Source: CAD feature listing. Evaluate the final solid. Frame: model axes, mm. Face numbers are marked on the shaded views. A direction names the side the tool comes from. Coordinates: 2 decimals unless noted, no trailing zeros. Order: outer loops, then holes, each group sorted by start corner. A loop starts at its lowest first (then second) coordinate and runs counter-clockwise, first axis right, second up.
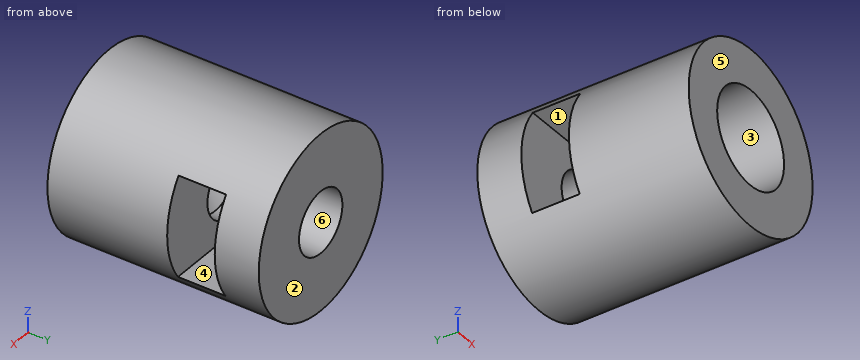
```python
from build123d import *

# Parameters (mm, degrees)
F3_R     = 5
F4_DEPTH = 12
F6_D     = 5.4
F6_DEPTH = 3
F6_TIP   = 1.6223236714
F7_D     = 3.5
F7_DEPTH = 6
F7_TIP   = 1.0515060833
F8_W     = 2.7
F8_H     = 5.7
F9_DEPTH = 38.4228628705


with BuildPart() as f4:
    # F3 (on Front) → F4 (new body)
    with BuildSketch(Plane.XZ):
        with Locations((-33.4218628705, 28.5066645592)):
            Circle(F3_R)
    extrude(amount=-F4_DEPTH)

    # F6
    with Locations(Plane.XZ):
        with Locations((-33.4218628705, 28.5066645592)):
            Hole(F6_D / 2, depth=F6_DEPTH)
            with Locations((0, 0, -(F6_DEPTH + F6_TIP / 2))):  # 118° drill point
                Cone(0, F6_D / 2, F6_TIP, mode=Mode.SUBTRACT)

    # F7
    with Locations(Plane(origin=(0, 12, 0), x_dir=(-1, 0, 0), z_dir=(0, 1, 0))):
        with Locations((33.4218628705, 28.5066645592)):
            Hole(F7_D / 2, depth=F7_DEPTH)
            with Locations((0, 0, -(F7_DEPTH + F7_TIP / 2))):  # 118° drill point
                Cone(0, F7_D / 2, F7_TIP, mode=Mode.SUBTRACT)

    # F8 (on Right) → F9 (cut, through all)
    with BuildSketch(Plane.YZ):
        with Locations((8.15, 28.5412482917)):
            Rectangle(F8_W, F8_H)
    extrude(amount=-F9_DEPTH, mode=Mode.SUBTRACT)


solid = f4.part
```
1. Ray query, line 1 (Z direction, x = -33.5, y = 10.5); line 2 (Y direction, x = -29.25, z = 29.25); line 3 (Z direction, x = -33.5, y = 8). Return the intervals inside material, ascending.
Findings:
line 1: z = 23.51 to 26.76, 30.25 to 33.51
line 2: y = 0 to 6.8, 9.5 to 12
line 3: z = 23.51 to 25.69, 31.39 to 33.51
2. Draft query along Y for the marked faces 4, 5 and 6. Return one class per face: released by +Y, released by -Y, zero draft, split by the parting line, or undercut.
Findings:
face 4: undercut
face 5: released by -Y
face 6: zero draft
3. Section query D-D on y = 11. Return loops of the section in (x, z), plus the area to 3 significant figures.
Findings:
outline: circle Ø10 at (-33.42, 28.51); hole circle Ø3.5 at (-33.42, 28.51)
area: 68.9 mm2
4. Section query C-C on z = 29.25. Count the separate pieces of the cut face and the enclosed holes in it, plus the area to 3 significant figures.
Findings:
separate pieces: 3
enclosed holes: 0
area: 61.2 mm2
5. Access query for the marked faces 1, 2 and 3. Directions: +Z, -Z, +X, -X, +Y, -Y. A direction counts if a zero-diameter tool reaches every point of the face in a straight line with its end or side. Return the directions, or none.
Findings:
face 1: +X, -X
face 2: +Z, -Z, +X, -X, +Y
face 3: -Y
6. Pin query (flat end, axial travel): P1, Ø3, axis at x = -36, y = 7.5, coming from the +Z side; P2, Ø1.7, axis at x = -32, z = 29.5, coming from the -Y side; P3, Ø3, axis at x = -33.42, z = 28.51, coming from the +Y side. Return the tip coordinate at first contact, or that it passes through.
Findings:
P1: stops at z = 33.39
P2: stops at y = 3.07
P3: stops at y = 5.85
7. Section query B-B on x = -37. Return loops of the section in (y, z).
Findings:
outline: (0, 25.01) - (12, 25.01) - (12, 32) - (0, 32) - close; hole (6.8, 25.69) - (9.5, 25.69) - (9.5, 31.39) - (6.8, 31.39) - close
8. Section query A-A on y = 8.75. Return loops of the section in (x, z), plus the area to 3 significant figures.
Findings:
outline: (-37.55, 25.69) arc R5 ccw to (-29.29, 25.69) - close; (-37.51, 31.39) - (-29.34, 31.39) arc R5 ccw to start
area: 24.8 mm2
